Geometry: see drawing. Coordinates: mm, zero at the bounding-box minimum. Coordinates: 2 decimals unless noted, no trailing zeros. Order: outer loops, then holes, each group sorted by start corner. A loop starts at its lowest first (then second) coordinate and runs counter-clockwise, first axis right, second up. Notation, with made-up numbers: (28.5, 21.25) -> (61.5, 21.25) arc R30 ccw to (61.5, 59.25) -> close; hole circle Ø3 at (-29.75, -16). An arc over 180 degrees is marked (long way). Use one line per item in the form item = value.
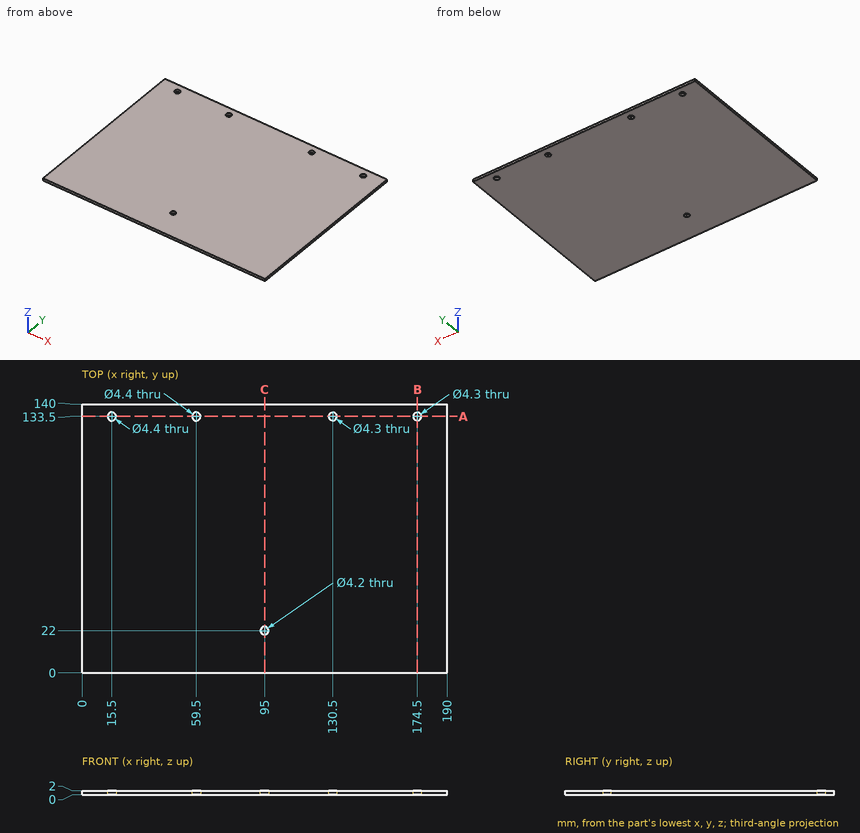
1) Section B-B, the plane x = 174.5. Output: boundary loops of the cut face in (y, z).
Results found:
outline = (0, 0) -> (131.35, 0) -> (131.35, 2) -> (0, 2) -> close; (135.65, 0) -> (140, 0) -> (140, 2) -> (135.65, 2) -> close
2) Section C-C, the plane x = 95. Output: boundary loops of the cut face in (y, z), and give its area (3 significant figures).
Results found:
outline = (0, 0) -> (19.9, 0) -> (19.9, 2) -> (0, 2) -> close; (24.1, 0) -> (140, 0) -> (140, 2) -> (24.1, 2) -> close
area = 272 mm2
3) Material intervals for probe 1 along X at (y, z) = (133.5, 0.5); probe 2 along Y at (x, z) = (59.5, 0.65); probe 3 along Y at (x, z) = (174.5, 1.05), sorted ascending. Write a range as from..to.
Results found:
probe_1 = 0..13.3, 17.7..57.3, 61.7..128.35, 132.65..172.35, 176.65..190
probe_2 = 0..131.3, 135.7..140
probe_3 = 0..131.35, 135.65..140
4) Section A-A, the plane y = 133.5. Output: boundary loops of the cut face in (x, z), and give its area (3 significant figures).
Results found:
outline = (0, 0) -> (13.3, 0) -> (13.3, 2) -> (0, 2) -> close; (17.7, 0) -> (57.3, 0) -> (57.3, 2) -> (17.7, 2) -> close; (61.7, 0) -> (128.35, 0) -> (128.35, 2) -> (61.7, 2) -> close; (132.65, 0) -> (172.35, 0) -> (172.35, 2) -> (132.65, 2) -> close; (176.65, 0) -> (190, 0) -> (190, 2) -> (176.65, 2) -> close
area = 345 mm2
